Input: dimensioned drawing with shaded views. Units: mm. Origin: part minimum x, y, z. Round coordinates to 2 decimals unless told otherwise and drop trailing zeros. Loops run counter-clockwise (first coordinate to the right, second up) from the corner with the lowest first, then second, coordinate; pieces in that order, holes last. Notation, with made-up numbers: (-17, 2.5) - (14, 2.5) arc R30 ccw to (14, 30.5) - close; hole circle Ø3 at (-35.5, 50). An arc over 180 degrees is marked (long way). Answer as CSV lines item,"result".
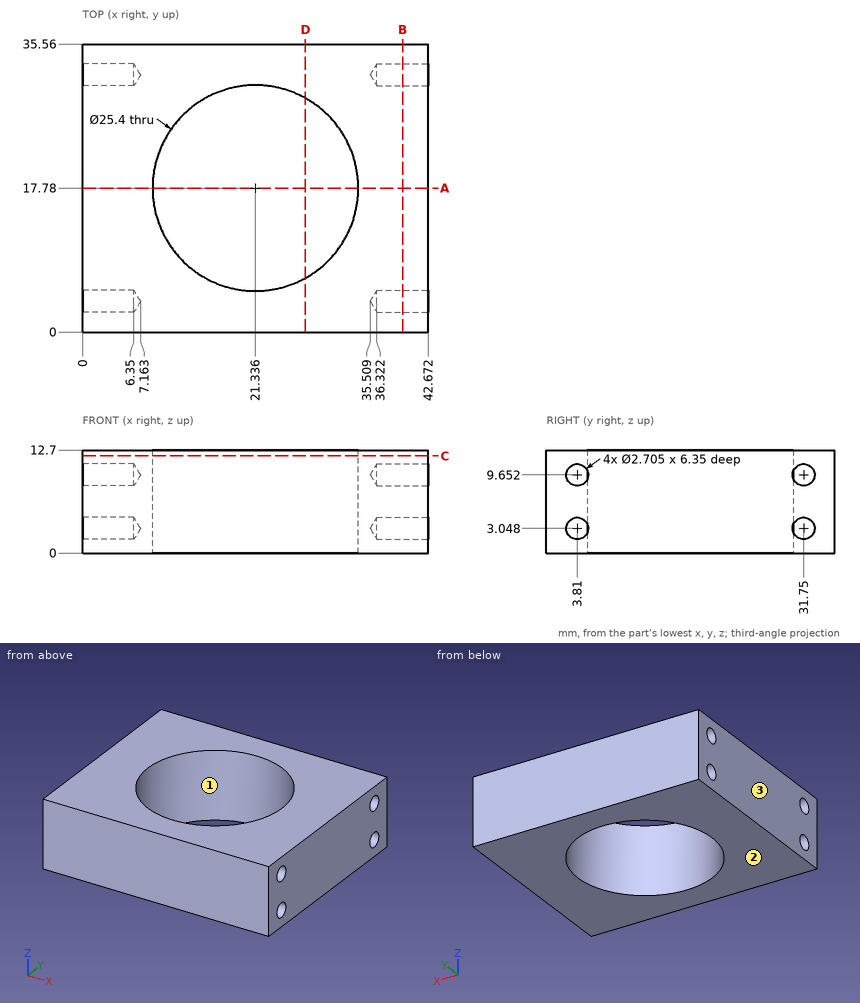
(1) Section A-A (y = 17.78). Output: boundary loops of the cut face in (x, z), and give its area (3 significant figures).
Findings below:
outline,"(0, 0) - (8.64, 0) - (8.64, 12.7) - (0, 12.7) - close; (34.04, 0) - (42.67, 0) - (42.67, 12.7) - (34.04, 12.7) - close"
area,"219 mm2"
(2) Section D-D (x = 27.5). Output: boundary loops of the cut face in (y, z).
Findings below:
outline,"(0, 0) - (6.68, 0) - (6.68, 12.7) - (0, 12.7) - close; (28.88, 0) - (35.56, 0) - (35.56, 12.7) - (28.88, 12.7) - close"
(3) Pin query (flat end, axial travel): P1, Ø2.5, axis at y = 3.81, z = 9.652, coming from the +X side; P2, Ø2.5, axis at y = 31.75, z = 9.652, coming from the -X side. Return the tip coordinate at first contact, or that it passes through.
Findings below:
P1,"x = 36.26"
P2,"x = 6.41"
(4) Section B-B (x = 39.5). Give the number of separate pieces and of enclosed holes in the cut face, and give its area (3 significant figures).
Findings below:
separate pieces,"1"
enclosed holes,"4"
area,"429 mm2"
(5) Draft query along X for the marked faces 1, 2 and 3. Return one class per face: pulls with the +X half, pulls with the -X half, needs draft (parallel to the pull), parting line crosses it, or undercut.
Findings below:
face 1,"undercut"
face 2,"needs draft"
face 3,"pulls with the -X half"
(6) Material intervals for line 1 along Z through (x, y) = (39.5, 3.81) (1 decimal); line 2 along Z through (x, y) = (1, 3) (1 decimal); line 3 along Y through (x, z) = (5, 8.5), sorted ascending.
Findings below:
line 1,"0 to 1.7, 4.4 to 8.3, 11 to 12.7"
line 2,"0 to 2, 4.1 to 8.6, 10.7 to 12.7"
line 3,"0 to 3.1, 4.52 to 31.04, 32.46 to 35.56"
(7) Section C-C (z = 12). Output: boundary loops of the cut face in (x, y).
Findings below:
outline,"(0, 0) - (42.67, 0) - (42.67, 35.56) - (0, 35.56) - close; hole circle Ø25.4 at (21.34, 17.78)"
